from build123d import *

# Parameters (mm, degrees)
F0_R     = 1.5
F0_R_2   = 11.1125
F1_DEPTH = 5.842
F3_DEPTH = 5.842
F5_DEPTH = 25.4
F6_R     = 2.363
F7_DEPTH = 25.4


with BuildPart() as f1:
    # F0 (on Front) → F1 (new body)
    with BuildSketch(Plane.XZ):
        Polygon((22.225, 22.225), (-22.225, 22.225), (-22.225, 19.05), (-28.067, 19.05), (-28.067, 6.35), (-22.225, 6.35), (-22.225, 1.7526), (-19.05, 1.7526), (-19.05, 3.048), (-15.875, 3.048), (-15.875, 1.7526), (-14.2875, 1.7526), (-14.2875, -1.7526), (-15.875, -1.7526), (-15.875, -3.048), (-19.05, -3.048), (-19.05, -1.7526), (-22.225, -1.7526), (-22.225, -6.35), (-28.067, -6.35), (-28.067, -19.05), (-22.225, -19.05), (-22.225, -22.225), (22.225, -22.225), (22.225, -19.05), (28.067, -19.05), (28.067, -6.35), (22.225, -6.35), (22.225, -1.7526), (19.05, -1.7526), (19.05, -3.048), (15.875, -3.048), (15.875, -1.7526), (14.2875, -1.7526), (14.2875, 1.7526), (15.875, 1.7526), (15.875, 3.048), (19.05, 3.048), (19.05, 1.7526), (22.225, 1.7526), (22.225, 6.35), (28.067, 6.35), (28.067, 19.05), (22.225, 19.05), align=None)
        with Locations((-15.5, -15.5)):
            Circle(F0_R, mode=Mode.SUBTRACT)
        with Locations((15.5, -15.5)):
            Circle(F0_R, mode=Mode.SUBTRACT)
        with Locations((-15.5, 15.5)):
            Circle(F0_R, mode=Mode.SUBTRACT)
        Circle(F0_R_2, mode=Mode.SUBTRACT)
        with Locations((15.5, 15.5)):
            Circle(F0_R, mode=Mode.SUBTRACT)
    extrude(amount=F1_DEPTH)

    # F2 (on face) → F3 (join, through all)
    with BuildSketch(Plane.XZ.offset(5.842)):
        Polygon((22.225, -22.225), (-22.225, -22.225), (-22.225, -31.75), (-28.067, -31.75), (-28.067, -44.45), (-22.225, -44.45), (-22.225, -47.625), (22.225, -47.625), (22.225, -44.45), (28.067, -44.45), (28.067, -31.75), (22.225, -31.75), align=None)
    extrude(amount=-F3_DEPTH)

    # F4 (on face) → F5 (cut)
    with BuildSketch(Plane(origin=(0, 0, 0), x_dir=(-1, 0, 0), z_dir=(0, 1, 0))):
        Polygon((22.225, -27.1526), (22.225, -23.6474), (19.05, -23.6474), (19.05, -22.352), (15.875, -22.352), (15.875, -23.6474), (12.7, -23.6474), (12.7, -27.1526), (15.875, -27.1526), (15.875, -28.448), (19.05, -28.448), (19.05, -27.1526), align=None)
        Polygon((-22.225, -27.1526), (-19.05, -27.1526), (-19.05, -28.448), (-15.875, -28.448), (-15.875, -27.1526), (-12.7, -27.1526), (-12.7, -23.6474), (-15.875, -23.6474), (-15.875, -22.352), (-19.05, -22.352), (-19.05, -23.6474), (-22.225, -23.6474), align=None)
    extrude(amount=-F5_DEPTH, mode=Mode.SUBTRACT)

    # F6 (on face) → F7 (cut)
    with BuildSketch(Plane.XZ.offset(5.842)):
        with Locations((-12.7, -36.957)):
            Circle(F6_R)
        with Locations((12.7, -36.957)):
            Circle(F6_R)
    extrude(amount=-F7_DEPTH, mode=Mode.SUBTRACT)


solid = f1.part
CAD build for the part. Positions are in the model's coordinates, mm. A direction names the side the tool comes from. Coordinates: 2 decimals unless noted, no trailing zeros. Order: outer loops, then holes, each group sorted by start corner. A loop starts at its lowest first (then second) coordinate and runs counter-clockwise, first axis right, second up.
Item 1: Band-saw the part on B-B on y = -2.3. Give the number of separate pieces and of enclosed holes in the cut face, plus the area to 3 significant figures.
Check sheet entries:
separate pieces: 1
enclosed holes: 7
area: 2,940 mm2
Item 2: Band-saw the part on A-A on x = -1.5. List the corners of the cut face in (y, z) (3 decimals).
Check sheet entries:
outline: (-5.842, -47.625) - (0, -47.625) - (0, -11.011) - (-5.842, -11.011) - close; (-5.842, 11.011) - (0, 11.011) - (0, 22.225) - (-5.842, 22.225) - close
Item 3: Drill centre lines: L1, parallel to Z at x = 21, y = -2.4 (3 decimals); L2, parallel to X at y = -2, z = -35.5; L3, parallel to Z at x = 17.5, y = -0.65 (3 decimals). Where is each one in solid material? Low to high.
Check sheet entries:
L1: z = -47.625 to -27.153, -23.647 to -1.753, 1.753 to 22.225
L2: x = -28.07 to -14.56, -10.84 to 10.84, 14.56 to 28.07
L3: z = -47.625 to -28.448, -22.352 to -3.048, 3.048 to 22.225
Item 4: 3-axis set-ups, long thin cutter, end or side, ignore diameter. For faces 4 (the face through (-22.225, -3, -46)), 5 (the face through (22.225, -3, 21)), 6 (the face through (14, -3, -23.647)), 7 (the face through (-17, -3, -28.448)), 8 (the face through (-21, -3, -1.753)): which of +Z, -Z, +X, -X, +Y, -Y reach the whole face in a straight line?
Check sheet entries:
face 4: -Z, -X, +Y, -Y
face 5: +Z, +X, +Y, -Y
face 6: +X, +Y, -Y
face 7: +Y, -Y
face 8: -X, +Y, -Y
Item 5: Two-plate mould, pull along Z, no slides. Class faces 1 (the face through (-17, -2.88, -15.43)), 2 (the face through (-28.067, -3, -38)), 3 (the face through (25, -3, 19.05)): +Z half, -Z half, draft (parallel to the pull), parting line (faces both ways), or undercut.
Check sheet entries:
face 1: undercut
face 2: draft
face 3: +Z half
Item 6: Pin check, flat tips, straight feed: pin 1 Ø1 at (y, z) = (-2, 2) entering from +X (3 decimals); pin 2 Ø1 at (y, z) = (-4.5, -2.5) entering from -X (3 decimals); pin 3 Ø2 at (x, z) = (6.5, -18) entering from +Y; pin 4 Ø3 at (x, y) = (-24.5, -4) entering from -Z. Stop position of each tip, or through.
Check sheet entries:
pin 1: stops at x = 22.225
pin 2: stops at x = -22.225
pin 3: stops at y = 0
pin 4: stops at z = -44.45
